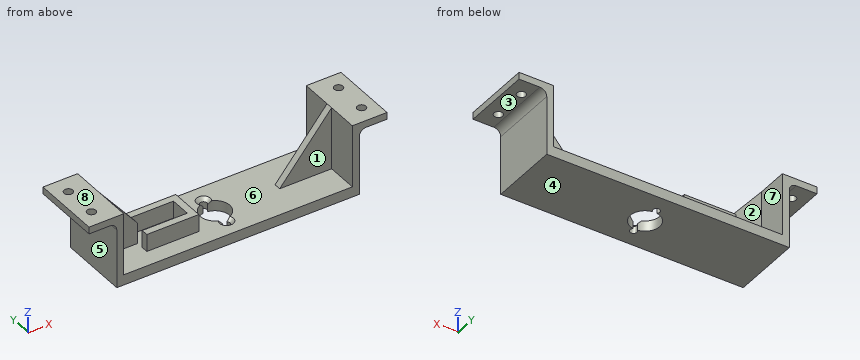
Autodesk Inventor part; units mm, degrees
ref_plane "Plano de trabajo1" through (-48.5042, -32, 20) normal (0, 0, -1) x (0, 1, 0)
ref_plane "XZ Plane" through (0, 0, 0) normal (0, 1, 0) x (-1, 0, 0)
ref_plane "XY Plane" through (0, 0, 0) normal (0, 0, 1) x (1, 0, 0)
sketch "Boceto1" plane through (0, 0, 0) normal (0, 0, 1) x (1, 0, 0)
  circle A0 centre (0, 0) radius 4.25
  line L0 (-35, -10) -> (35, -10)
  line L1 (35, -10) -> (35, 10)
  line L2 (35, 10) -> (-35, 10)
  line L3 (-35, 10) -> (-35, -10)
  line L4 (-35, -10) -> (35, 10) construction
  line L5 (35, -10) -> (-35, 10) construction
  circle A1 centre (0, 0) radius 8
  dimension "d0" = 8.5
  dimension "d1" = 70
  dimension "d2" = 20
  dimension "d3" = 16
extrude "Extrusión1" add sketch "Boceto1" along normal blind 3 contours L3 L2 L1 L0 | A1
sketch "Boceto3" plane through (0, 0, 3) normal (0, 0, 1) x (1, 0, 0)
  line L0 (-35, 10) -> (-35, -10)
  line L1 (-35, -10) -> (-33, -10)
  line L2 (-33, -10) -> (-33, 10)
  line L3 (-33, 10) -> (-35, 10)
  line L4 (-35, 10) -> (-35, -10)
  line L5 (35, -10) -> (33, -10)
  line L6 (33, -10) -> (33, 10)
  line L7 (33, 10) -> (35, 10)
  line L8 (35, 10) -> (35, -10)
  point P0 (0, 0)
  dimension "d10" = 2
  dimension "d11" = 20
  dimension "d12" = 2
  dimension "d13" = 20
ref_plane "Plano de trabajo1" through (-48.5042, -32, 20) normal (0, 0, -1) x (0, 1, 0)
extrude "Extrusión3" add sketch "Boceto3" along normal blind 18
sketch "Boceto4" plane through (0, 0, 3) normal (0, 0, 1) x (1, 0, 0)
  circle A0 centre (0, 0) radius 4.25
  circle A1 centre (0, -5) radius 1
  circle A2 centre (0, 5) radius 1
hole "Agujero1" at (0, -5, 3) at (0, 5, 3) direction (0, 0, -1) diameter 2 depth 3
chamfer "Chaflán1" distance 1 angle 45 2 edges at (0, -6, 3) (0, 6, 3)
sketch "Boceto5" plane through (-35, -10, 0) normal (-1, 0, 0) x (0, 0, 1)
  line L0 (0, 0) -> (21, 0)
  line L1 (21, 0) -> (19, 0)
  line L2 (19, 0) -> (19, 20)
  line L3 (19, 20) -> (21, 20)
  line L4 (21, 20) -> (21, 0)
  point P0 (0, 10)
  dimension "d49" = 2
  dimension "d50" = 20
extrude "Extrusión4" add sketch "Boceto5" along normal blind 8
sketch "Boceto6" plane through (35, -10, 0) normal (1, 0, 0) x (0, 0, -1)
  line L0 (0, 20) -> (-21, 20)
  line L1 (-21, 20) -> (-19, 20)
  line L2 (-19, 20) -> (-19, 0)
  line L3 (-19, 0) -> (-21, 0)
  line L4 (-21, 0) -> (-21, 20)
  point P0 (0, 10)
  dimension "d51" = 2
  dimension "d52" = 20
extrude "Extrusión5" add sketch "Boceto6" along normal blind 8
sketch "Boceto8" plane through (0, 0, 21) normal (0, 0, 1) x (1, 0, 0)
  line L0 (43, 10) -> (43, -10)
  line L1 (33, 10) -> (43, 10)
  line L2 (33, -10) -> (43, -10)
  point P0 (0, 0)
  point P1 (39, -5)
  point P2 (39, 5)
  dimension "d53" = 4
  dimension "d54" = 4
  dimension "d55" = 5
  dimension "d56" = 5
hole "Agujero3" at (39, 5, 21) at (39, -5, 21) direction (0, 0, -1) diameter 2.5 end through all
sketch "Boceto9" plane through (0, 0, 21) normal (0, 0, 1) x (1, 0, 0)
  line L0 (-33, 10) -> (-43, 10)
  line L1 (-43, -10) -> (-43, 10)
  line L2 (-33, -10) -> (-43, -10)
  point P0 (0, 0)
  point P1 (-39, 5)
  point P2 (-39, -5)
  dimension "d64" = 5
  dimension "d65" = 4
  dimension "d73" = 5
  dimension "d74" = 4
hole "Agujero4" at (-39, 5, 21) at (-39, -5, 21) direction (0, 0, -1) diameter 2.5 end through all
sketch "Boceto10" plane through (0, 0, 3) normal (0, 0, 1) x (1, 0, 0)
  line L0 (33, -10) -> (33, 10)
  line L1 (33, 0) -> (33, 1)
  line L2 (33, 0) -> (34, 0) construction
  line L3 (33, 1) -> (18, 1)
  line L4 (18, 1) -> (18, -1)
  line L5 (18, -1) -> (33, -1)
  line L6 (33, -1) -> (33, 1)
  point P0 (0, 0)
  dimension "d75" = 1
  dimension "d76" = 90
  dimension "d77" = 15
  dimension "d78" = 2
extrude "Extrusión6" add sketch "Boceto10" along normal blind 18
chamfer "Chaflán2" distance 15 distance2 18 1 edges at (18, 0, 21) measured on face at (42.0563, 1.5189, 21)
fillet "Empalme2" radius 2 2 edges at (35, 0, 19) (-35, 0, 19)
mirror "Simetría1" about plane through (0, 0, 0) normal (1, 0, 0) of "Extrusión6", "Chaflán2"
ref_plane "Plano de trabajo2" through (-10, 0, 0) normal (1, 0, 0) x (0, 1, 0)
sketch "Boceto12" plane through (0, 0, 3) normal (0, 0, 1) x (1, 0, 0)
  line L0 (-10, -3) -> (-21, -3)
  line L1 (-21, -3) -> (-21, 3)
  line L2 (-10, 3) -> (-21, 3)
  line L3 (-10, -3) -> (-10, 3)
  point P0 (0, 0)
extrude "Extrusión7" cut sketch "Boceto12" along normal blind 10
sketch "Boceto13" plane through (0, 0, 3) normal (0, 0, 1) x (1, 0, 0)
  line L0 (-10, -3) -> (-21, -3)
  line L1 (-21, -3) -> (-21, 3)
  line L2 (-10, 3) -> (-21, 3)
  line L3 (-10, -3) -> (-10, 3)
  line L4 (-23, -5) -> (-8, -5)
  line L5 (-8, -5) -> (-8, 5)
  line L6 (-8, 5) -> (-23, 5)
  line L7 (-23, 5) -> (-23, -5)
  line L8 (-10, -3) -> (-8, -3)
  line L9 (-10, 3) -> (-8, 3)
  line L10 (-33, -1) -> (-21, -1)
  line L11 (-21, 1) -> (-33, 1)
  line L12 (-21, -3) -> (-23, -3)
  line L13 (-21, 3) -> (-23, 3)
  point P0 (0, 0)
  point P1 (-23, 1)
  point P2 (-23, -1)
  dimension "d88" = 2
extrude "Extrusión8" add sketch "Boceto13" along normal blind 5 contours L8 L5 L4 L7 L12 L0 | L3 L9 L5 L8 | L2 L13 L7 L6 L5 L9 | L10 L7 L11 L1
sketch "Boceto14" plane through (0, 0, 8) normal (0, 0, 1) x (1, 0, 0)
  line L0 (-10, 3) -> (-23, 3)
  line L1 (-23, -3) -> (-10, -3)
  line L2 (-10, 3) -> (-23, 3)
  line L3 (-23, 3) -> (-23, -3)
  line L4 (-23, -3) -> (-10, -3)
  line L5 (-10, -3) -> (-10, 3)
  point P0 (0, 0)
extrude "Extrusión9" cut sketch "Boceto14" along normal blind 5 and the other way blind 5
properties part number "Soporte motor"
Could you check a few things on this model? Use its own coordinates, in mm. Face numbers are marked on the shaded views. A direction names the side the tool comes from. Coordinates: 2 decimals unless noted, no trailing zeros. Write each loop counter-clockwise with the first axis right and the second up, starting at its lowest first coordinate (ties: lowest second). Pieces come first, ordered by that corner, then holes. Notation, with made-up numbers: (-8, -31.5) - (40, -31.5) arc R28 ccw to (40, 4.5) - close; hole circle Ø8 at (11, 62.5). An arc over 180 degrees is marked (long way). Use a Markdown table: item, result.
Q1. Imagine slicing it at C-C (x = -14). List the corners of the cut face in (y, z) for me, and give its area (3 significant figures).
Geometry check:
| item | result |
|---|---|
| outline | (-10, 0) - (10, 0) - (10, 3) - (5, 3) - (5, 8) - (3, 8) - (3, 3) - (-3, 3) - (-3, 8) - (-5, 8) - (-5, 3) - (-10, 3) - close |
| area | 80.0 mm2 |
Q2. I'm going to push flat-ended pins straight in: pin 1 Ø10 at (y, z) = (5.5, 7.5) entering from +X; pin 2 Ø1.5 at (x, y) = (23, 1) entering from +Z; pin 3 Ø1.5 at (x, y) = (-19, 7) entering from +Z. Where does each tip first touch, or does it pass through?
Geometry check:
| item | result |
|---|---|
| pin 1 | stops at x = 35 |
| pin 2 | stops at z = 9.9 |
| pin 3 | stops at z = 3 |
Q3. Imagine slicing it at B-B (z = 4.25). List the corners of the cut face in (x, y) for me, and give its area (3 significant figures).
Geometry check:
| item | result |
|---|---|
| outline | (-35, -10) - (-33, -10) - (-33, -1) - (-23, -1) - (-23, 1) - (-33, 1) - (-33, 10) - (-35, 10) - close; (-23, -5) - (-8, -5) - (-8, 5) - (-23, 5) - (-23, 3) - (-10, 3) - (-10, -3) - (-23, -3) - close; (19.04, -1) - (33, -1) - (33, -10) - (35, -10) - (35, 10) - (33, 10) - (33, 1) - (19.04, 1) - close |
| area | 200 mm2 |
Q4. Imagine slicing it at D-D (z = 14). List the corners of the cut face in (x, y) for me.
Geometry check:
| item | result |
|---|---|
| outline | (-35, -10) - (-33, -10) - (-33, -1) - (-27.17, -1) - (-27.17, 1) - (-33, 1) - (-33, 10) - (-35, 10) - close; (27.17, -1) - (33, -1) - (33, -10) - (35, -10) - (35, 10) - (33, 10) - (33, 1) - (27.17, 1) - close |
Q5. Imagine slicing it at A-A (x = 39). List the corners of the cut face in (y, z) for me.
Geometry check:
| item | result |
|---|---|
| outline | (-10, 19) - (-6.25, 19) - (-6.25, 21) - (-10, 21) - close; (-3.75, 19) - (3.75, 19) - (3.75, 21) - (-3.75, 21) - close; (6.25, 19) - (10, 19) - (10, 21) - (6.25, 21) - close |
Q6. Thinking about a two-plate mould opening in X: for the marked faces 5, 6, 7 and 8, which applies, +X half, -X half, draft (parallel to the pull), parting line (faces both ways), or undercut?
Geometry check:
| item | result |
|---|---|
| face 5 | -X half |
| face 6 | undercut |
| face 7 | undercut |
| face 8 | draft |
Q7. Which directions (+Z, -Z, +X, -X, +Y, -Y) give clear straight access to the entire face, cutting with the end or side of a thin tool? Please do the marked faces 1, 2, 3 and 4.
Geometry check:
| item | result |
|---|---|
| face 1 | +Z, -Y |
| face 2 | +Z, +Y |
| face 3 | -Z, +X, +Y, -Y |
| face 4 | -Z, +X, -X, +Y, -Y |
Q8. Please list where these lines run through material, in increasing order: L1, parallel to Y at x = 39, z = 20.3; L2, parallel to X at y = -5, z = 19.7; L3, parallel to X at y = 1.5, z = 16.5.
Geometry check:
| item | result |
|---|---|
| L1 | y = -10 to -6.25, -3.75 to 3.75, 6.25 to 10 |
| L2 | x = -43 to -40.25, -37.75 to -33, 33 to 37.75, 40.25 to 43 |
| L3 | x = -35 to -33, 33 to 35 |
